```python
from build123d import *

# Parameters (mm, degrees)
BOSS_EXTRUDE1_DEPTH     = 3.81
CUT_EXTRUDE1_DEPTH      = 18.281637299
CIRPATTERN1_COUNT       = 6
MIRROR1_COPY_1_DEPTH    = 18.281637299
MIRROR1_COPY_2_DEPTH    = 18.281637299
MIRROR1_COPY_3_DEPTH    = 18.281637299
MIRROR1_COPY_4_DEPTH    = 18.281637299
MIRROR1_COPY_5_DEPTH    = 18.281637299
CUT_EXTRUDE2_DEPTH      = 19.498737463
CUT_EXTRUDE2_DEPTH_BACK = 19.498737463


with BuildPart() as part:
    # Sketch1 → Boss-Extrude1 (new, symmetric)
    with BuildSketch(Plane.XY):
        with BuildLine():
            Line((-5.026722801, 5.910971637), (-7.407741623, 6.593717798))
            ThreePointArc((-7.407741623, 6.593717798), (-8.766513969, 6.679662371), (-10.036356458, 6.18859332))
            ThreePointArc((-10.036356458, 6.18859332), (-10.13048223, 6.088494289), (-10.170107647, 5.956929464))
            ThreePointArc((-10.170107647, 5.956929464), (-9.960464677, 4.611679084), (-9.20664832, 3.477920001))
            Line((-9.20664832, 3.477920001), (-7.424863389, 1.757270295))
            ThreePointArc((-7.424863389, 1.757270295), (-7.270818157, 1.595014723), (-7.131420667, 1.420014312))
            ThreePointArc((-7.131420667, 1.420014312), (-6.637662134, -0.097259644), (-7.131420667, -1.6145336))
            ThreePointArc((-7.131420667, -1.6145336), (-7.270818157, -1.789534012), (-7.424863389, -1.951789584))
            Line((-7.424863389, -1.951789584), (-9.20664832, -3.67243929))
            ThreePointArc((-9.20664832, -3.67243929), (-9.960464677, -4.806198373), (-10.170107647, -6.151448752))
            ThreePointArc((-10.170107647, -6.151448752), (-10.13048223, -6.283013578), (-10.036356458, -6.383112608))
            ThreePointArc((-10.036356458, -6.383112608), (-8.766513969, -6.87418166), (-7.407741623, -6.788237086))
            Line((-7.407741623, -6.788237086), (-5.026722801, -6.105490926))
            ThreePointArc((-5.026722801, -6.105490926), (-4.809182738, -6.053211627), (-4.587929191, -6.019990065))
            ThreePointArc((-4.587929191, -6.019990065), (-3.027052134, -6.351019611), (-1.95993361, -7.537264021))
            ThreePointArc((-1.95993361, -7.537264021), (-1.878077553, -7.745485994), (-1.814582722, -7.960020865))
            Line((-1.814582722, -7.960020865), (-1.215348831, -10.363416732))
            ThreePointArc((-1.215348831, -10.363416732), (-0.610392842, -11.583120388), (0.449806676, -12.437301716))
            ThreePointArc((0.449806676, -12.437301716), (0.583557866, -12.468767511), (0.717309055, -12.437301716))
            ThreePointArc((0.717309055, -12.437301716), (1.777508573, -11.583120388), (2.382464562, -10.363416732))
            Line((2.382464562, -10.363416732), (2.981698454, -7.960020865))
            ThreePointArc((2.981698454, -7.960020865), (3.045193285, -7.745485994), (3.127049342, -7.537264021))
            ThreePointArc((3.127049342, -7.537264021), (4.194167866, -6.351019611), (5.755044922, -6.019990065))
            ThreePointArc((5.755044922, -6.019990065), (5.976298469, -6.053211627), (6.193838533, -6.105490926))
            Line((6.193838533, -6.105490926), (8.574857355, -6.788237086))
            ThreePointArc((8.574857355, -6.788237086), (9.933629701, -6.87418166), (11.203472189, -6.383112608))
            ThreePointArc((11.203472189, -6.383112608), (11.297597962, -6.283013578), (11.337223379, -6.151448752))
            ThreePointArc((11.337223379, -6.151448752), (11.127580408, -4.806198373), (10.373764051, -3.67243929))
            Line((10.373764051, -3.67243929), (8.591979121, -1.951789584))
            ThreePointArc((8.591979121, -1.951789584), (8.437933888, -1.789534012), (8.298536398, -1.6145336))
            ThreePointArc((8.298536398, -1.6145336), (7.804777866, -0.097259644), (8.298536398, 1.420014312))
            ThreePointArc((8.298536398, 1.420014312), (8.437933888, 1.595014723), (8.591979121, 1.757270295))
            Line((8.591979121, 1.757270295), (10.373764051, 3.477920001))
            ThreePointArc((10.373764051, 3.477920001), (11.127580408, 4.611679084), (11.337223379, 5.956929464))
            ThreePointArc((11.337223379, 5.956929464), (11.297597962, 6.088494289), (11.203472189, 6.18859332))
            ThreePointArc((11.203472189, 6.18859332), (9.933629701, 6.679662371), (8.574857355, 6.593717798))
            Line((8.574857355, 6.593717798), (6.193838533, 5.910971637))
            ThreePointArc((6.193838533, 5.910971637), (5.976298469, 5.858692338), (5.755044922, 5.825470777))
            ThreePointArc((5.755044922, 5.825470777), (4.194167866, 6.156500322), (3.127049342, 7.342744732))
            ThreePointArc((3.127049342, 7.342744732), (3.045193285, 7.550966706), (2.981698454, 7.765501576))
            Line((2.981698454, 7.765501576), (2.382464562, 10.168897443))
            ThreePointArc((2.382464562, 10.168897443), (1.777508573, 11.3886011), (0.717309055, 12.242782428))
            ThreePointArc((0.717309055, 12.242782428), (0.583557866, 12.274248223), (0.449806676, 12.242782428))
            ThreePointArc((0.449806676, 12.242782428), (-0.610392842, 11.3886011), (-1.215348831, 10.168897443))
            Line((-1.215348831, 10.168897443), (-1.814582722, 7.765501576))
            ThreePointArc((-1.814582722, 7.765501576), (-1.878077553, 7.550966706), (-1.95993361, 7.342744732))
            ThreePointArc((-1.95993361, 7.342744732), (-3.027052134, 6.156500322), (-4.587929191, 5.825470777))
            ThreePointArc((-4.587929191, 5.825470777), (-4.809182738, 5.858692338), (-5.026722801, 5.910971637))
        make_face()
    extrude(amount=BOSS_EXTRUDE1_DEPTH, both=True)

    # Sketch2 → Cut-Extrude1 (cut, symmetric)
    with BuildSketch(Plane(origin=(0, 0, 0), x_dir=(0, 0, -1), z_dir=(1, 0, 0))):
        Polygon((-3.048, 12.274248223), (-3.81, 7.765501576), (-3.81, 12.274248223), align=None)
    cut_extrude1 = extrude(amount=CUT_EXTRUDE1_DEPTH, both=True, mode=Mode.SUBTRACT)

    # CirPattern1: Cut-Extrude1 ×6 about axis
    cirpattern1_axis = Axis((0.583557866, -0.097259644, 0), (0, 0, 1))
    for i in range(1, CIRPATTERN1_COUNT):
        add(cut_extrude1.rotate(cirpattern1_axis, i * 360 / CIRPATTERN1_COUNT), mode=Mode.SUBTRACT)

    # Mirror1: Cut-Extrude1 across plane
    add(cut_extrude1.mirror(Plane.XY), mode=Mode.SUBTRACT)

    # Mirror1 copy 1 sketch → Mirror1 copy 1 (cut, symmetric)
    with BuildSketch(Plane(origin=(0.20754961, -0.554005758, 0), x_dir=(0, 0, 1), z_dir=(0.5000000000000001, 0.8660254037844386, 0))):
        Polygon((-3.048, -12.274248223), (-3.81, -7.765501576), (-3.81, -12.274248223), align=None)
    extrude(amount=MIRROR1_COPY_1_DEPTH, both=True, mode=Mode.SUBTRACT)

    # Mirror1 copy 2 sketch → Mirror1 copy 2 (cut, symmetric)
    with BuildSketch(Plane(origin=(0.791107476, -0.651265403, 0), x_dir=(0, 0, 1), z_dir=(-0.4999999999999998, 0.8660254037844387, 0))):
        Polygon((-3.048, -12.274248223), (-3.81, -7.765501576), (-3.81, -12.274248223), align=None)
    extrude(amount=MIRROR1_COPY_2_DEPTH, both=True, mode=Mode.SUBTRACT)

    # Mirror1 copy 3 sketch → Mirror1 copy 3 (cut, symmetric)
    with BuildSketch(Plane(origin=(1.167115731, -0.194519289, 0), x_dir=(0, 0, 1), z_dir=(-1, 0, 0))):
        Polygon((-3.048, -12.274248223), (-3.81, -7.765501576), (-3.81, -12.274248223), align=None)
    extrude(amount=MIRROR1_COPY_3_DEPTH, both=True, mode=Mode.SUBTRACT)

    # Mirror1 copy 4 sketch → Mirror1 copy 4 (cut, symmetric)
    with BuildSketch(Plane(origin=(0.959566121, 0.35948647, 0), x_dir=(0, 0, 1), z_dir=(-0.5000000000000004, -0.8660254037844384, 0))):
        Polygon((-3.048, -12.274248223), (-3.81, -7.765501576), (-3.81, -12.274248223), align=None)
    extrude(amount=MIRROR1_COPY_4_DEPTH, both=True, mode=Mode.SUBTRACT)

    # Mirror1 copy 5 sketch → Mirror1 copy 5 (cut, symmetric)
    with BuildSketch(Plane(origin=(0.376008256, 0.456746114, 0), x_dir=(0, 0, 1), z_dir=(0.5000000000000001, -0.8660254037844386, 0))):
        Polygon((-3.048, -12.274248223), (-3.81, -7.765501576), (-3.81, -12.274248223), align=None)
    extrude(amount=MIRROR1_COPY_5_DEPTH, both=True, mode=Mode.SUBTRACT)

    # Sketch3 → Cut-Extrude2 (cut, two sides: drawn at the far end of the back side and taken through both)
    with BuildSketch(Plane(origin=(0, 0, -3.81), x_dir=(-1, 0, 0), z_dir=(0, 0, -1)).offset(-CUT_EXTRUDE2_DEPTH_BACK)):
        Polygon((1.249529239, -3.272259644), (3.082616344, -0.097259644), (1.249529239, 3.077740356), (-2.41664497, 3.077740356), (-4.249732075, -0.097259644), (-2.41664497, -3.272259644), align=None)
    extrude(amount=CUT_EXTRUDE2_DEPTH + CUT_EXTRUDE2_DEPTH_BACK, mode=Mode.SUBTRACT)


solid = part.part
```
Here's how the part is built. I have some questions about the finished solid (model axes, mm). A direction names the side the tool comes from. Give positions to 0.01 mm unless a question says otherwise; leave off trailing zeros. Order: outer loops, then holes, each group sorted by start corner. A loop starts at its lowest first (then second) coordinate and runs counter-clockwise, first axis right, second up. Notation, with made-up numbers: (2.5, -33.5) - (37.5, -33.5) arc R25 cw to (37.5, 2.5) - close; hole circle Ø10 at (47.25, 66.5). An arc over 180 degrees is marked (long way). Answer as a JSON object with one key per item and string values. Group by question number.
Item 1: If we section it at B-B on y = 4: Please give me the cut outline in (x, z).
Item 2: If we mould it in two halves opening along X, with no side actions, what happens to faces 5 (the flat face through (9, 4.7, -3.5)), 6 (the flat face through (0.5, -3.5, -3.81)), 7 (the flat face through (3.32, 1.51, 0.05))? For each: pulls with the +X half, pulls with the -X half, needs draft (parallel to the pull), parting line crosses it, or undercut.
Item 3: Which directions (+Z, -Z, +X, -X, +Y, -Y) give clear straight access to the entire face, cutting with the end or side of a thin tool? Please do faces 1 (the flat face through (-6.201, 6.248, 0.053)), 2 (the flat face through (9.495, -2.824, 0.053)), 3 (the flat face through (-2.15, -1.71, 0.05)), 4 (the flat face through (-8.303, -2.8, 0.053)).
Item 4: If we section it at D-D on x = 3.5: Please give me the cut outline in (y, z).
Item 5: If we section it at A-A on x = 10: Please give me the cut outline in (y, z), and give its area (3 significant figures).
Item 6: If we section it at C-C on x = -5.5: Please give me the cut outline in (y, z).
Item 7: For P1, Ø2, axis at x = -1, y = 2.5, coming from the -Z side; P2, Ø1, axis at x = -8, z = -1.5, coming from the -Y side; P3, Ø1.5, axis at x = 7, z = -1.5, coming from the +Y side; P4, Ø3, axis at y = -3, z = 2.5, coming from the +X side, each with a flat end and sliding along its axis, tell me the tip position at first contact or that it passes through.
Item 8: Please list where these lines run through material, in increasing order: probe 1 along Y at (x, z) = (9.5, -2); probe 2 along Y at (x, z) = (-6, -2); probe 3 along X at (y, z) = (2.25, 0.5).
Result set:
{
 "1": {"outline": "(-9.64, -3.3) - (-6.13, -3.81) - (7.3, -3.81) - (10.81, -3.3) - (10.81, 3.3) - (7.3, 3.81) - (-6.13, 3.81) - (-9.64, 3.3) - close"},
 "2": {"face 5": "pulls with the +X half", "face 6": "needs draft", "face 7": "undercut"},
 "3": {"face 1": "+Z, -Z, +Y", "face 2": "+Z, -Z, +X", "face 3": "+Z, -Z", "face 4": "+Z, -Z, -X"},
 "4": {"outline": "(-6.94, -3.81) - (-1.4, -3.81) - (-1.4, 3.81) - (-6.94, 3.81) - close; (1.2, -3.81) - (6.74, -3.81) - (6.74, 3.81) - (1.2, 3.81) - close"},
 "5": {"outline": "(-6.86, -3.19) - (-3.31, -3.49) - (-3.31, 3.49) - (-6.86, 3.19) - close; (3.12, -3.49) - (6.67, -3.19) - (6.67, 3.19) - (3.12, 3.49) - close", "area": "47.4 mm²"},
 "6": {"outline": "(-6.24, -3.73) - (-5.29, -3.81) - (5.09, -3.81) - (6.05, -3.73) - (6.05, 3.73) - (5.09, 3.81) - (-5.29, 3.81) - (-6.24, 3.73) - close"},
 "7": {"P1": "z = -3.81", "P2": "y = -6.91", "P3": "y = 6.36", "P4": "x = 10.99"},
 "8": {"probe 1": "-6.91 to -2.83, 2.63 to 6.72", "probe 2": "-6.38 to 6.19", "probe 3": "-7.94 to -1.73, 2.89 to 9.1"}
}
